Autodesk Inventor part; units mm, degrees
ref_plane "YZ Plane" through (0, 0, 0) normal (1, 0, 0) x (0, 1, 0)
ref_plane "XZ Plane" through (0, 0, 0) normal (0, 1, 0) x (-1, 0, 0)
ref_plane "XY Plane" through (0, 0, 0) normal (0, 0, 1) x (1, 0, 0)
sketch "Sketch1" plane through (0, 0, 0) normal (0, 0, 1) x (1, 0, 0)
  line L0 (0, 0) -> (152.4, 0)
  line L1 (152.4, 0) -> (152.4, 101.6)
  line L2 (152.4, 101.6) -> (0, 101.6)
  line L3 (0, 101.6) -> (0, 0)
  circle A0 centre (38.1, 50.8) radius 3.5
  circle A1 centre (63.5, 50.8) radius 3.5
  circle A2 centre (88.9, 50.8) radius 3.5
  circle A3 centre (114.3, 50.8) radius 3.5
  circle A4 centre (50.8, 76.2) radius 2.5
  circle A5 centre (76.2, 76.2) radius 2.5
  circle A6 centre (101.6, 76.2) radius 2.5
  line L4 (12.7, 101.6) -> (25.4, 101.6)
  line L5 (25.4, 101.6) -> (25.4, 97.6)
  line L6 (25.4, 97.6) -> (12.7, 97.6)
  line L7 (12.7, 97.6) -> (12.7, 101.6)
  line L8 (139.7, 101.6) -> (127, 101.6)
  line L9 (127, 101.6) -> (127, 97.6)
  line L10 (127, 97.6) -> (139.7, 97.6)
  line L11 (139.7, 97.6) -> (139.7, 101.6)
  line L12 (139.7, 0) -> (127, 0)
  line L13 (127, 0) -> (127, 4)
  line L14 (127, 4) -> (139.7, 4)
  line L15 (139.7, 4) -> (139.7, 0)
  line L16 (12.7, 0) -> (25.4, 0)
  line L17 (25.4, 0) -> (25.4, 4)
  line L18 (25.4, 4) -> (12.7, 4)
  line L19 (12.7, 4) -> (12.7, 0)
  line L20 (0, 57.15) -> (4, 57.15)
  line L21 (4, 57.15) -> (4, 44.45)
  line L22 (4, 44.45) -> (0, 44.45)
  line L23 (0, 44.45) -> (0, 57.15)
  line L24 (152.4, 57.15) -> (148.4, 57.15)
  line L25 (148.4, 57.15) -> (148.4, 44.45)
  line L26 (148.4, 44.45) -> (152.4, 44.45)
  line L27 (152.4, 44.45) -> (152.4, 57.15)
  point P0 (76.2, 0)
  point P1 (76.2, 101.6)
  point P2 (12.7, 99.6)
  point P3 (139.7, 99.6)
  point P4 (12.7, 2)
  point P5 (0, 50.8)
  point P6 (4, 50.8)
  point P7 (148.4, 50.8)
  point P8 (152.4, 50.8)
  point P9 (0, 50.8)
  dimension "d0" = 152.4
  dimension "d1" = 101.6
  dimension "d2" = 7
  dimension "d5" = 25.4
  dimension "d10" = 12.7
  dimension "d11" = 50.8
  dimension "d12" = 5
  dimension "d15" = 25.4
  dimension "d20" = 25.4
  dimension "d21" = 12.7
  dimension "d22" = 4
  dimension "d23" = 12.7
  dimension "d24" = 12.7
  dimension "d25" = 4
  dimension "d26" = 12.7
  dimension "d27" = 4
  dimension "d28" = 12.7
  dimension "d29" = 4
  dimension "d30" = 4
  dimension "d31" = 12.7
  dimension "d32" = 4
  dimension "d33" = 12.7
  dimension "d34" = 12.7
  dimension "d35" = 12.7
extrude "Extrusion1" add sketch "Sketch1" along normal blind 4 contours L3 L22 L21 L20 L2 L7 L6 L5 L9 L10 L11 L1 L24 L25 L26 L0 L15 L14 L13 L17 L18 L19
properties part number "Front Panel" material "Wood (Birch)"
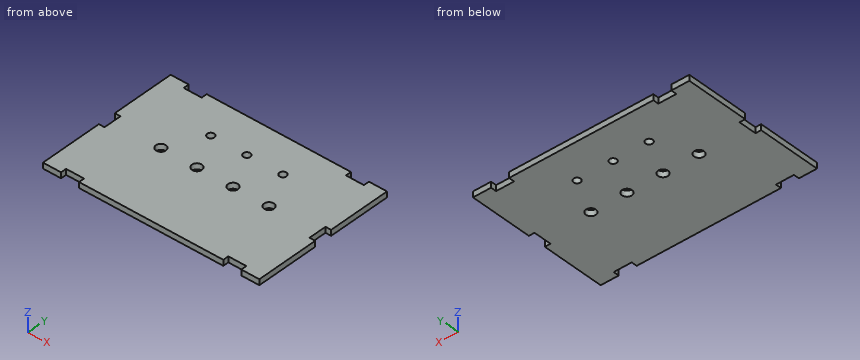
Check sheet for the modelled part. Datum: model origin and axes. Units: mm. Give positions to 0.01 mm unless a question says otherwise; leave off trailing zeros. Write each loop counter-clockwise with the first axis right and the second up, starting at its lowest first coordinate (ties: lowest second). Pieces come first, ordered by that corner, then holes.
Item 1: Cross-section at A-A (x = 50.8). Enter the section's corners in (y, z), and give its area (3 significant figures).
Item 2: Cross-section at D-D (z = 2.75). Count the separate pieces of the cut face and the enclosed holes in it, and give its area (3 significant figures).
Item 3: Scan lines: L1, parallel to Y at x = 114.5, z = 2.95; L2, parallel to Y at x = 101.6, z = 1.3; L3, parallel to X at y = 77.5, z = 3.1. Record each from-to range of solid material in increasing order.
Item 4: Gauge pin test, flat ends, axial feed: pin 1 (2 mm diameter, centred on y = 99, z = 1.5, fed in from -X); pin 2 (2 mm diameter, centred on y = 56, z = 3, fed in from -X); pin 3 (1.2 mm diameter, centred on x = 22, z = 2, fed in from +Y). Record the tip position at first contact, or that the pin passes through.
Item 5: Cross-section at B-B (y = 76.2). Enter the section's corners in (x, z), and give its area (3 significant figures).
Item 6: Cross-section at C-C (x = 114.3). Enter the section's corners in (y, z), and give its area (3 significant figures).
Report:
1. outline: (0, 0) - (73.7, 0) - (73.7, 4) - (0, 4) - close; (78.7, 0) - (101.6, 0) - (101.6, 4) - (78.7, 4) - close
1. area: 386 mm2
2. separate pieces: 1
2. enclosed holes: 7
2. area: 15,000 mm2
3. L1: y = 0 to 47.31, 54.29 to 101.6
3. L2: y = 0 to 73.7, 78.7 to 101.6
3. L3: x = 0 to 48.66, 52.94 to 74.06, 78.34 to 99.46, 103.74 to 152.4
4. pin 1: stops at x = 0
4. pin 2: stops at x = 4
4. pin 3: stops at y = 97.6
5. outline: (0, 0) - (48.3, 0) - (48.3, 4) - (0, 4) - close; (53.3, 0) - (73.7, 0) - (73.7, 4) - (53.3, 4) - close; (78.7, 0) - (99.1, 0) - (99.1, 4) - (78.7, 4) - close; (104.1, 0) - (152.4, 0) - (152.4, 4) - (104.1, 4) - close
5. area: 550 mm2
6. outline: (0, 0) - (47.3, 0) - (47.3, 4) - (0, 4) - close; (54.3, 0) - (101.6, 0) - (101.6, 4) - (54.3, 4) - close
6. area: 378 mm2
